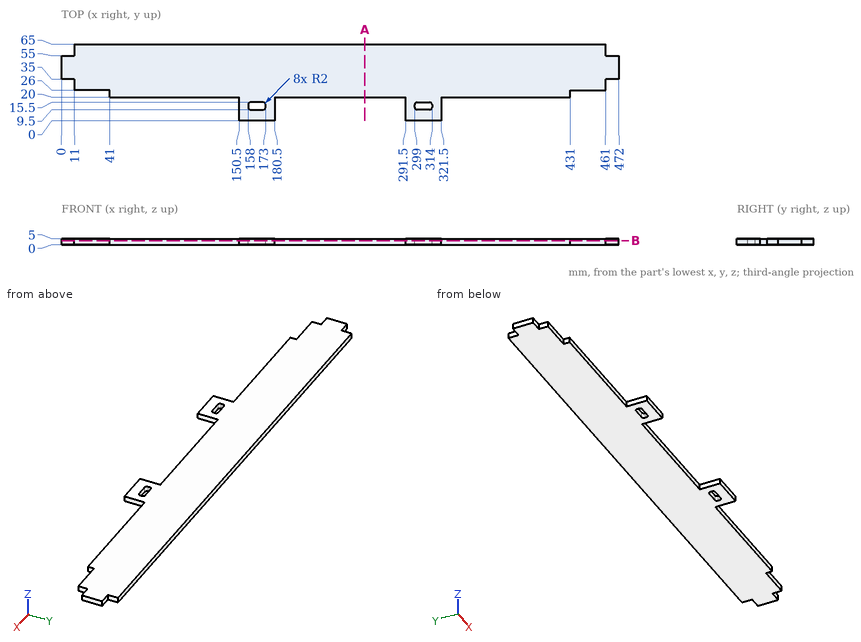
Could you check a few things on this drawing? It's one solid part, dimensions in mm from its lowest x, y, z. Round coordinates to 2 decimals unless told otherwise and drop trailing zeros. Order: outer loops, then holes, each group sorted by start corner. A loop starts at its lowest first (then second) coordinate and runs counter-clockwise, first axis right, second up.
(1) I'm going to push flat-ended pins straight in: pin 1 (3 mm diameter, centred on y = 13.5, z = 3.5, fed in from +X); pin 2 (1 mm diameter, centred on y = 12.5, z = 2, fed in from -X); pin 3 (2.5 mm diameter, centred on y = 31.5, z = 3, fed in from -X). Where does each tip first touch, or does it pass through?
Response values:
pin 1: stops at x = 321.5
pin 2: stops at x = 150.5
pin 3: stops at x = 11
(2) Imagine slicing it at A-A (x = 257). Write out the boundary of the cut face in (y, z), plus the area to 3 significant figures.
Response values:
outline: (20, 0) - (65, 0) - (65, 5) - (20, 5) - close
area: 225 mm2
(3) Imagine slicing it at B-B (z = 3.5). Count the separate pieces of the cut face and the enclosed holes in it, plus the area to 3 significant figures.
Response values:
separate pieces: 1
enclosed holes: 2
area: 21,400 mm2
(4) Please list where these lines run through material, in increasing order: line 1 along X through (y, z) = (13, 1.45); line 2 along Y through (x, z) = (165.5, 1.1); line 3 along X through (y, z) = (10, 3.8).
Response values:
line 1: x = 150.5 to 158, 173 to 180.5, 291.5 to 299, 314 to 321.5
line 2: y = 0 to 9.5, 15.5 to 65
line 3: x = 150.5 to 158.68, 172.32 to 180.5, 291.5 to 299.68, 313.32 to 321.5
